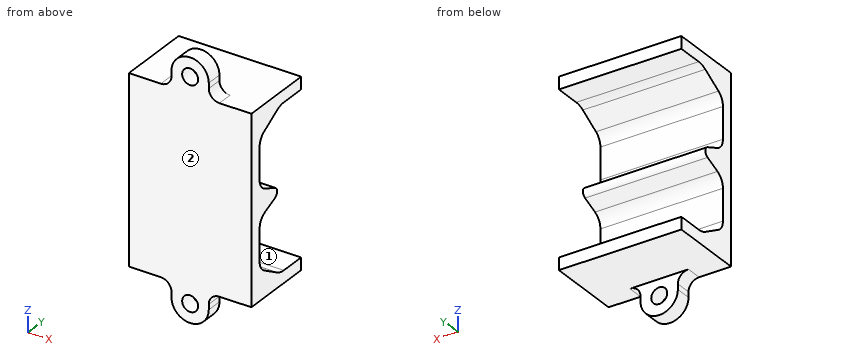
Autodesk Inventor part; units mm, degrees
ref_plane "YZ Plane" through (0, 0, 0) normal (1, 0, 0) x (0, 1, 0)
ref_plane "XZ Plane" through (0, 0, 0) normal (0, 1, 0) x (-1, 0, 0)
ref_plane "XY Plane" through (0, 0, 0) normal (0, 0, 1) x (1, 0, 0)
sketch "Sketch1" plane through (0, 0, 0) normal (1, 0, 0) x (0, 1, 0)
  arc A0 (-7.974, 10.8816) -> (-8.874, 9.3228) centre (-7.074, 9.3228) ccw
  line L0 (-8.874, 9.3228) -> (-8.874, 3.4133)
  line L1 (-8.874, 9.3228) -> (-8.874, 3.4133)
  arc A1 (-1.981, -0.7039) -> (0, -1) centre (-0.4181, 2.9781) ccw
  line L2 (-7.7773, 1.7564) -> (-1.981, -0.7039)
  line L3 (2.1178, 13.4219) -> (-2.7701, 13.4219)
  line L4 (-1.981, -0.7039) -> (2.1178, 13.4219)
  line L5 (2.1178, 13.4219) -> (-2.7701, 13.4219)
  arc A2 (-2.7701, 13.4219) -> (-4.2701, 13.02) centre (-2.7701, 10.4219) ccw
  line L6 (-4.2701, 13.02) -> (-12.9304, 8.02)
  line L7 (-4.2701, 13.02) -> (-7.974, 10.8816)
  circle A3 centre (-7.074, 9.3228) radius 1.8
  circle A4 centre (-2.7701, 10.4219) radius 3
  arc A5 (-8.874, 3.4133) -> (-7.7773, 1.7564) centre (-7.074, 3.4133) ccw
  circle A6 centre (-7.074, 3.4133) radius 1.8
  line L8 (0, -1) -> (-3.8233, -1)
  arc A7 (-8.874, -11.3228) -> (-7.974, -12.8816) centre (-7.074, -11.3228) ccw
  line L9 (-8.874, -11.3228) -> (-8.874, -5.4133)
  line L10 (-8.874, -11.3228) -> (-8.874, -5.4133)
  line L11 (-7.7773, -3.7564) -> (-1.981, -1.2961)
  line L12 (2.1178, -15.4219) -> (-2.7701, -15.4219)
  line L13 (-1.981, -1.2961) -> (2.1178, -15.4219)
  line L14 (2.1178, -15.4219) -> (-2.7701, -15.4219)
  arc A8 (-4.2701, -15.02) -> (-2.7701, -15.4219) centre (-2.7701, -12.4219) ccw
  line L15 (-4.2701, -15.02) -> (-12.9304, -10.02)
  line L16 (-4.2701, -15.02) -> (-7.974, -12.8816)
  circle A9 centre (-7.074, -11.3228) radius 1.8
  circle A10 centre (-2.7701, -12.4219) radius 3
  arc A11 (-7.7773, -3.7564) -> (-8.874, -5.4133) centre (-7.074, -5.4133) ccw
  circle A12 centre (-7.074, -5.4133) radius 1.8
  line L17 (-1.981, -0.7039) -> (-1.981, -1.2961)
  line L18 (2.1178, 13.4219) -> (2.1178, 16.4219)
  line L19 (2.1178, 16.4219) -> (-11.8822, 16.4219)
  line L20 (-11.8822, 16.4219) -> (-11.8822, -18.4221)
  line L21 (-11.8822, -18.4221) -> (2.1178, -18.4221)
  line L22 (2.1178, -18.4221) -> (2.1178, -15.4219)
  point P0 (0, 0)
  point P1 (4.8736, 0.62)
  point P2 (-0.4181, -4.9781)
  point P3 (-4.2701, -15.02)
  point P4 (-7.974, 10.8816)
  dimension "d0" = 10
  dimension "d1" = 3
  dimension "d2" = 14
  dimension "d3" = 34.844
extrude "Extrusion1" add sketch "Sketch1" along normal blind 23 contours L6 L20 L19 L18 L3 A2 | A0 L0 A5 L2 L17 L11 A11 L9 A7 L15 L20 L6 | L15 A8 L12 L22 L21 L20
sketch "Sketch2" plane through (23, 0, 0) normal (1, 0, 0) x (0, 0, -1)
  line L0 (-13.4219, -2.7701) -> (-13.4219, 2.1178)
  line L1 (-13.4219, 2.1178) -> (-13.4219, -2.7701)
  line L2 (-13.4219, -2.7701) -> (-14.1219, -2.7701)
  line L3 (-14.1219, -2.7701) -> (-14.1219, 2.1178)
  line L4 (-14.1219, 2.1178) -> (-13.4219, 2.1178)
  line L5 (-10.8816, -7.974) -> (-13.02, -4.2701)
  line L6 (-13.02, -4.2701) -> (-10.8816, -7.974)
  line L7 (-10.8816, -7.974) -> (-11.4878, -8.324)
  line L8 (-11.4878, -8.324) -> (-13.6262, -4.6201)
  line L9 (-13.6262, -4.6201) -> (-13.02, -4.2701)
  arc A0 (-10.8816, -7.974) -> (-9.3228, -8.874) centre (-9.3228, -7.074) ccw
  arc A1 (-3.4133, -8.874) -> (-1.7564, -7.7773) centre (-3.4133, -7.074) ccw
  line L10 (-9.3228, -8.874) -> (-3.4133, -8.874)
  line L11 (-3.4133, -8.874) -> (-3.4133, -9.574)
  line L12 (-3.4133, -9.574) -> (-9.3228, -9.574)
  line L13 (-9.3228, -9.574) -> (-9.3228, -8.874)
  line L14 (0.7039, -1.981) -> (-1.7564, -7.7773)
  line L15 (-1.7564, -7.7773) -> (0.7039, -1.981)
  line L16 (0.7039, -1.981) -> (1.3483, -2.2546)
  line L17 (1.3483, -2.2546) -> (-1.1121, -8.0508)
  line L18 (-1.1121, -8.0508) -> (-1.7564, -7.7773)
  line L19 (1.2961, -1.981) -> (0.7039, -1.981)
  line L20 (1, -1.981) -> (1, -3.9334)
  arc A2 (-13.4219, -2.7701) -> (-13.02, -4.2701) centre (-10.4219, -2.7701) ccw
  circle A3 centre (-10.4219, -2.7701) radius 3.7
  circle A4 centre (-9.3228, -7.074) radius 2.5
  circle A5 centre (-3.4133, -7.074) radius 2.5
  line L21 (15.4219, -2.7701) -> (15.4219, 2.1178)
  line L22 (15.4219, 2.1178) -> (15.4219, -2.7701)
  line L23 (15.4219, -2.7701) -> (16.1219, -2.7701)
  line L24 (16.1219, -2.7701) -> (16.1219, 2.1178)
  line L25 (16.1219, 2.1178) -> (15.4219, 2.1178)
  line L26 (12.8816, -7.974) -> (15.02, -4.2701)
  line L27 (15.02, -4.2701) -> (12.8816, -7.974)
  line L28 (12.8816, -7.974) -> (13.4878, -8.324)
  line L29 (13.4878, -8.324) -> (15.6262, -4.6201)
  line L30 (15.6262, -4.6201) -> (15.02, -4.2701)
  arc A6 (11.3228, -8.874) -> (12.8816, -7.974) centre (11.3228, -7.074) ccw
  arc A7 (3.7564, -7.7773) -> (5.4133, -8.874) centre (5.4133, -7.074) ccw
  line L31 (11.3228, -8.874) -> (5.4133, -8.874)
  line L32 (5.4133, -8.874) -> (5.4133, -9.574)
  line L33 (5.4133, -9.574) -> (11.3228, -9.574)
  line L34 (11.3228, -9.574) -> (11.3228, -8.874)
  line L35 (1.2961, -1.981) -> (3.7564, -7.7773)
  line L36 (3.7564, -7.7773) -> (1.2961, -1.981)
  line L37 (0.6517, -2.2546) -> (3.1121, -8.0508)
  line L38 (3.1121, -8.0508) -> (3.7564, -7.7773)
  arc A8 (15.02, -4.2701) -> (15.4219, -2.7701) centre (12.4219, -2.7701) ccw
  circle A9 centre (12.4219, -2.7701) radius 3.7
  circle A10 centre (11.3228, -7.074) radius 2.5
  circle A11 centre (5.4133, -7.074) radius 2.5
  point P0 (0, 0)
  point P1 (13.7491, -6.4715)
  point P2 (13.6826, -6.2487)
  point P3 (13.9372, -6.1456)
  point P4 (-11.9372, -6.1456)
  point P5 (-11.6826, -6.2487)
  point P6 (-11.7491, -6.4715)
  point P7 (-13.6262, -4.6201)
  point P8 (-9.3228, -9.574)
  point P9 (-1.1121, -8.0508)
  point P10 (1, -3.0751)
  point P11 (3.1121, -8.0508)
  point P12 (11.3228, -9.574)
  point P13 (15.6262, -4.6201)
  point P14 (16.1219, -2.7701)
  point P15 (15.4219, -0.6045)
  point P16 (9.6476, -5.2182)
  point P17 (9.5878, -8.874)
  point P18 (7.1483, -8.874)
  point P19 (3.0785, -6.1803)
  point P20 (-1.0785, -6.1803)
  point P21 (-5.1483, -8.874)
  point P22 (-7.5878, -8.874)
  point P23 (-7.6476, -5.2182)
  point P24 (-13.4219, -0.6045)
  point P25 (-14.1219, -2.7701)
  dimension "d6" = 0.7
  dimension "d7" = 0.7
  dimension "d8" = 0.7
  dimension "d9" = 0.7
extrude "Extrusion2" cut sketch "Sketch2" against normal blind 23 contours L2 A3 L0 | A2 L9 A3 L2 | L0 A3 A4 L5 A2 | A3 L3 L4 L0 | L5 A3 L9 | A3 L5 A4 L8 | A4 L10 A0 L5 A3 | A3 A4 | A4 L5 L7 | L7 A0 L13 A4 | A4 L10 A5 L12 | L13 L10 A4 | A5 L10 L11 | L11 A1 L18 A5 | A5 L14 A1 L10 | A5 L14 L16 L20 L17 | L18 L14 A5 | L20 L16 L17 | L17 L16 L20 L19 L35 A11 L37 | L19 L20 L16 | A11 L35 L38 | L38 A7 L32 A11 | L35 A11 L31 A7 | A11 L31 A10 L33 | L32 L31 A11 | A10 L31 L34 | L34 A6 L28 A10 | L31 A10 A9 L26 A6 | A10 L26 A9 L29 | L28 L26 A10 | A9 L26 L30 | L30 A8 L23 A9 | A10 A9 | A9 L21 A8 L26 A10 | A9 L21 L25 L24 | L23 L21 A9
fillet "Fillet1" radius 1 1 edges at (11.5, -3.0751, -1)
sketch "Sketch3" plane through (0, -11.8822, -18.4221) normal (0, -1, 0) x (1, 0, 0)
  line L0 (0, 0) -> (23, 0)
  line L1 (11.5, 0) -> (11.5, -3)
  line L2 (0, 34.844) -> (23, 34.844)
  line L3 (11.5, 34.844) -> (11.5, 37.844)
  circle A0 centre (11.5, 37.844) radius 1.5
  circle A1 centre (11.5, -3) radius 1.5
  line L4 (11.5, 37.844) -> (11.5, -3) construction
  line L5 (8, 37.844) -> (8, -3)
  line L6 (15, -3) -> (15, 37.844)
  arc A2 (15, 37.844) -> (8, 37.844) centre (11.5, 37.844) ccw
  arc A3 (8, -3) -> (15, -3) centre (11.5, -3) ccw
  point P0 (0, 18.4221)
  point P1 (11.5, 17.422)
  point P2 (8, 0)
  point P3 (15, 0)
  point P4 (15, 34.844)
  point P5 (8, 34.844)
  dimension "d13" = 3
  dimension "d14" = 3
  dimension "d15" = 3
  dimension "d16" = 3
  dimension "d17" = 7
extrude "Extrusion3" add sketch "Sketch3" against normal blind 3 contours L0 L6 A3 L5 | L5 A2 L6 L2
fillet "Fillet2" radius 2 4 edges at (15, -10.3822, 16.4219) (8, -10.3822, 16.4219) (15, -10.3822, -18.4221) (8, -10.3822, -18.4221)
properties part number "wago_support"
Design review of the part built by this model. Coordinates are the model's own, in mm. Face numbers are marked on the shaded views. A direction names the side the tool comes from. Round coordinates to 2 decimals unless told otherwise and drop trailing zeros. Loops run counter-clockwise (first coordinate to the right, second up) from the corner with the lowest first, then second, coordinate; pieces in that order, holes last. Notation, with made-up numbers: M 60,61 L 85,61 A19 cw 85,92 Z; hole C 55,4.25 d1. An arc over 180 degrees is marked long. Answer as a JSON object with one key per item and string values.
Item 1: We need section C-C on z = 8.5. Give the boundary of the cut face in (x, y), and give its area (3 significant figures).
Answer sheet:
{"outline": "M 0,-11.88 L 23,-11.88 L 23,-9.57 L 0,-9.57 Z", "area": "53.1 mm^2"}
Item 2: We need section B-B on x = 11.5. State how many separate pieces and enclosed holes the cut face has, and give its area (3 significant figures).
Answer sheet:
{"separate pieces": "3", "enclosed holes": "0", "area": "193 mm^2"}
Item 3: Clearance check with flat-ended pins moving along their axes: P1, Ø1, axis at x = 9.5, z = -4, coming from the +Y side; P2, Ø1.5, axis at x = 15.5, z = 6.5, coming from the +Y side; P3, Ø1.5, axis at x = 8, y = 0, coming from the -Z side; P4, Ø1.5, axis at y = -4.5, z = 13.5, coming from the -X side. State where each tip first meets the part, or that it passes through.
Answer sheet:
{"P1": "stops at y = -8.68", "P2": "stops at y = -9.57", "P3": "stops at z = -18.42", "P4": "stops at x = 0"}
Item 4: We need section D-D on x = 8.75. Give the boundary of the cut face in (y, z).
Answer sheet:
{"outline": "M -11.88,-23.59 L -8.88,-23.59 L -8.88,-18.42 L 2.12,-18.42 L 2.12,-16.12 L -2.77,-16.12 A3.7 cw -4.62,-15.63 L -8.32,-13.49 A2.5 cw -9.57,-11.32 L -9.57,-5.41 A2.5 cw -8.05,-3.11 L -5.24,-1.92 A1 ccw -5.24,-0.08 L -8.05,1.11 A2.5 cw -9.57,3.41 L -9.57,9.32 A2.5 cw -8.32,11.49 L -4.62,13.63 A3.7 cw -2.77,14.12 L 2.12,14.12 L 2.12,16.42 L -8.88,16.42 L -8.88,21.59 L -11.88,21.59 Z"}
Item 5: Machinability: for the marked faces 1 and 2, which of the approach directions +Z, -Z, +X, -X, +Y, -Y give a long, thin tool a straight path to every point of the face, cutting with its end or side? Answer none if there is none.
Answer sheet:
{"face 1": "+X, -X, +Y", "face 2": "+Z, -Z, +X, -X, -Y"}
Item 6: Wall thickness on L1, parallel to Z at x = 7.75, y = 0.25; L2, parallel to Z at x = 11.5, y = -9.65; L3, parallel to Z at x = 20.25, y = -5.25: over which ranges is each line inside the solid? List them lowest first. Write a range as from..to.
Answer sheet:
{"L1": "z = -18.42..-16.12, 14.12..16.42", "L2": "z = -24.92..-22.92, -19.92..17.92, 20.92..22.92", "L3": "z = -18.42..-15.26, -1.92..-0.08, 13.26..16.42"}
Item 7: We need section A-A on z = -22. Give the boundary of the cut face in (x, y), and give its area (3 significant figures).
Answer sheet:
{"outline": "M 8.05,-11.88 L 10.12,-11.88 L 10.12,-8.88 L 8.05,-8.88 Z; M 12.88,-11.88 L 14.95,-11.88 L 14.95,-8.88 L 12.88,-8.88 Z", "area": "12.4 mm^2"}
